from build123d import *

# Parameters (mm, degrees)
BOSS_EXTRUDE1_DEPTH = 12.7
FILLET1_R           = 10


with BuildPart() as part:
    # Sketch1 → Boss-Extrude1 (new body)
    with BuildSketch(Plane.XY):
        Polygon((307.625143269, 169.700104384), (325.725145069, 169.700104384), (325.725145069, -174.977895616), (-321.974854931, -174.977895616), (-321.974854931, 169.700104384), (-303.974854931, 169.700104384), (-303.974854931, 148.700104384), (-281.974854931, 148.700104384), (-281.974854931, 169.700104384), (285.625143269, 169.700104384), (285.625143269, 148.700104384), (307.625143269, 148.700104384), align=None)
        with BuildLine():
            Line((317.221591679, -169.977895616), (316.221591679, -169.977895616))
            ThreePointArc((316.221591679, -169.977895616), (314.453824726, -169.245662569), (313.721591679, -167.477895616))
            Line((313.721591679, -167.477895616), (313.721591679, -162.477895616))
            ThreePointArc((313.721591679, -162.477895616), (314.453824726, -160.710128663), (316.221591679, -159.977895616))
            Line((316.221591679, -159.977895616), (317.221591679, -159.977895616))
            ThreePointArc((317.221591679, -159.977895616), (318.989358632, -160.710128663), (319.721591679, -162.477895616))
            Line((319.721591679, -162.477895616), (319.721591679, -167.477895616))
            ThreePointArc((319.721591679, -167.477895616), (318.989358632, -169.245662569), (317.221591679, -169.977895616))
        make_face(mode=Mode.SUBTRACT)
        with BuildLine():
            Line((-312.778408321, -169.977895616), (-313.778408321, -169.977895616))
            ThreePointArc((-313.778408321, -169.977895616), (-315.546175274, -169.245662569), (-316.278408321, -167.477895616))
            Line((-316.278408321, -167.477895616), (-316.278408321, -162.477895616))
            ThreePointArc((-316.278408321, -162.477895616), (-315.546175274, -160.710128663), (-313.778408321, -159.977895616))
            Line((-313.778408321, -159.977895616), (-312.778408321, -159.977895616))
            ThreePointArc((-312.778408321, -159.977895616), (-311.010641368, -160.710128663), (-310.278408321, -162.477895616))
            Line((-310.278408321, -162.477895616), (-310.278408321, -167.477895616))
            ThreePointArc((-310.278408321, -167.477895616), (-311.010641368, -169.245662569), (-312.778408321, -169.977895616))
        make_face(mode=Mode.SUBTRACT)
        with BuildLine():
            Line((-312.674854931, 154.702104384), (-313.674854931, 154.702104384))
            ThreePointArc((-313.674854931, 154.702104384), (-315.442621884, 155.434337431), (-316.174854931, 157.202104384))
            Line((-316.174854931, 157.202104384), (-316.174854931, 162.202104384))
            ThreePointArc((-316.174854931, 162.202104384), (-315.442621884, 163.969871337), (-313.674854931, 164.702104384))
            Line((-313.674854931, 164.702104384), (-312.674854931, 164.702104384))
            ThreePointArc((-312.674854931, 164.702104384), (-310.907087978, 163.969871337), (-310.174854931, 162.202104384))
            Line((-310.174854931, 162.202104384), (-310.174854931, 157.202104384))
            ThreePointArc((-310.174854931, 157.202104384), (-310.907087978, 155.434337431), (-312.674854931, 154.702104384))
        make_face(mode=Mode.SUBTRACT)
        with BuildLine():
            Line((317.325145069, 154.702104384), (316.325145069, 154.702104384))
            ThreePointArc((316.325145069, 154.702104384), (314.557378116, 155.434337431), (313.825145069, 157.202104384))
            Line((313.825145069, 157.202104384), (313.825145069, 162.202104384))
            ThreePointArc((313.825145069, 162.202104384), (314.557378116, 163.969871337), (316.325145069, 164.702104384))
            Line((316.325145069, 164.702104384), (317.325145069, 164.702104384))
            ThreePointArc((317.325145069, 164.702104384), (319.092912022, 163.969871337), (319.825145069, 162.202104384))
            Line((319.825145069, 162.202104384), (319.825145069, 157.202104384))
            ThreePointArc((319.825145069, 157.202104384), (319.092912022, 155.434337431), (317.325145069, 154.702104384))
        make_face(mode=Mode.SUBTRACT)
    extrude(amount=BOSS_EXTRUDE1_DEPTH)

    # Fillet1
    fillet1_edges = [part.edges().sort_by_distance(p)[0] for p in [
        (-321.974854931, 169.700104384, 6.35),
        (-321.974854931, -174.977895616, 6.35),
        (325.725145069, -174.977895616, 6.35),
        (325.725145069, 169.700104384, 6.35),
    ]]
    fillet(fillet1_edges, radius=FILLET1_R)


solid = part.part
Check sheet for the modelled part. Datum: model origin and axes. Units: mm. A direction names the side the tool comes from. Round coordinates to 2 decimals unless told otherwise and drop trailing zeros.
1. Gauge pin test, flat ends, axial feed: pin 1 Ø4 at (x, z) = (-289.5, 7.5) entering from +Y; pin 2 Ø0.8 at (x, z) = (-313.5, 6) entering from +Y. Record the tip position at first contact, or that the pin passes through.
2. Set-up check for faces 1 (the flat face through (325.725, 0, 6)), 2 (the flat face through (-281.975, 159, 6)): record each of +Z, -Z, +X, -X, +Y, -Y from which the full face is reachable in a straight line by a thin tool's end or side.
3. Scan line: probe 1 along Y at (x, z) = (-290, 11.75). Record every from-to range of solid material in increasing order.
4. Mould release check, pull along X, two halves, no side actions. Record for faces 3 (the flat face through (-321.975, -5, 6)), 4 (the flat face through (-2, 169.7, 6)), 5 (the flat face through (-303.975, 159, 6)): released by +X, released by -X, zero draft, split by the parting line, or undercut.
Recorded:
1. pin 1: stops at y = 148.7
1. pin 2: stops at y = 169.64
2. face 1: +Z, -Z, +X, +Y, -Y
2. face 2: +Z, -Z, +Y
3. probe 1: y = -174.98 to 148.7
4. face 3: released by -X
4. face 4: zero draft
4. face 5: undercut
